from build123d import *

# Parameters (mm, degrees)
ESQUISSE1_W             = 100
ESQUISSE1_H             = 130
BOSS_EXTRU_1_DEPTH      = 6
ESQUISSE2_W             = 6
ESQUISSE2_H             = 30
ENL_V_MAT_EXTRU_1_DEPTH = 6


with BuildPart() as part:
    # Esquisse1 → Boss.-Extru.1 (new body)
    with BuildSketch(Plane.XY):
        with Locations((-50, 65)):
            Rectangle(ESQUISSE1_W, ESQUISSE1_H)
    extrude(amount=BOSS_EXTRU_1_DEPTH)

    # Esquisse2 → Enlèv. mat.-Extru.1 (cut)
    with BuildSketch(Plane.XY.offset(6)):
        Polygon((-100, 130), (-70, 130), (-70, 124), (-94, 124), (-94, 100), (-100, 100), align=None)
        Polygon((0, 130), (-30.235491659, 130), (-30.235491659, 124), (-6.235491659, 124), (-6.235491659, 100), (0, 100), align=None)
        Polygon((-100, 0), (-70, 0), (-70, 6), (-94, 6), (-94, 30), (-100, 30), align=None)
        Polygon((0, 0), (-30, 0), (-30, 6), (-6, 6), (-6, 30), (0, 30), align=None)
        with Locations((-97, 65)):
            Rectangle(ESQUISSE2_W, ESQUISSE2_H)
        with Locations((-3, 65)):
            Rectangle(ESQUISSE2_W, ESQUISSE2_H)
    extrude(amount=-ENL_V_MAT_EXTRU_1_DEPTH, mode=Mode.SUBTRACT)


solid = part.part
Read the model definition and answer for the solid it produces. Units are mm, in the model's axes. A direction names the side the tool comes from. Round coordinates to 2 decimals unless told otherwise and drop trailing zeros. Write each loop counter-clockwise with the first axis right and the second up, starting at its lowest first coordinate (ties: lowest second). Pieces come first, ordered by that corner, then holes. Notation, with made-up numbers: M 85.5,-20.5 L 134.5,-20.5 A15 ccw 134.5,-5.5 Z; hole C 5.5,65 d5. An arc over 180 degrees is marked long. Use a Markdown table: item, result.
1) Straight lines are drawn through the part: line 1 along Y through (x, z) = (-87, 4.15); line 2 along X through (y, z) = (108, 4.35); line 3 along X through (y, z) = (23.5, 5). For each, find the intervals that lie inside material, in ascending order. Write a range as [from, to].
Answers follow:
| item | result |
|---|---|
| line 1 | y = [6, 124] |
| line 2 | x = [-94, -6.24] |
| line 3 | x = [-94, -6] |
2) Flat-ended cylindrical pins translate along their axes: pin 1 (1.8 mm diameter, centred on x = -4.5, z = 3, fed in from -Y); pin 2 (1.8 mm diameter, centred on x = -21, z = 2.5, fed in from +Y); pin 3 (8 mm diameter, centred on x = -88.5, y = 63, fed in from -Z); pin 4 (1.8 mm diameter, centred on y = 107.5, z = 2.5, fed in from -X). Find the tip coordinate at first contact, or state that the pin passes through.
Answers follow:
| item | result |
|---|---|
| pin 1 | stops at y = 30 |
| pin 2 | stops at y = 124 |
| pin 3 | stops at z = 0 |
| pin 4 | stops at x = -94 |
3) For a pull along Y with two mould halves and no side action, classify faces 4 (the flat face through (0, 40, 3)), 5 (the flat face through (-18, 6, 3)), 6 (the flat face through (-6, 65, 3)) as pulls with the +Y half, pulls with the -Y half, needs draft (parallel to the pull), parting line crosses it, or undercut.
Answers follow:
| item | result |
|---|---|
| face 4 | needs draft |
| face 5 | pulls with the -Y half |
| face 6 | undercut |
4) The part is cut by section A-A (z = 4.5). Write down the section's boundary in (x, y).
Answers follow:
| item | result |
|---|---|
| outline | M -100,30 L -94,30 L -94,6 L -70,6 L -70,0 L -30,0 L -30,6 L -6,6 L -6,30 L 0,30 L 0,50 L -6,50 L -6,80 L 0,80 L 0,100 L -6.24,100 L -6.24,124 L -30.24,124 L -30.24,130 L -70,130 L -70,124 L -94,124 L -94,100 L -100,100 L -100,80 L -94,80 L -94,50 L -100,50 Z |
5) The part is cut by section C-C (x = -22.5). Write down the section's boundary in (y, z).
Answers follow:
| item | result |
|---|---|
| outline | M 6,0 L 124,0 L 124,6 L 6,6 Z |
6) The part is cut by section B-B (y = 52). Write down the section's boundary in (x, z).
Answers follow:
| item | result |
|---|---|
| outline | M -94,0 L -6,0 L -6,6 L -94,6 Z |
7) A tool of negligible diameter and unlimited length cuts with its end or side. For faces 1 (the flat face through (-30, 3, 3)), 2 (the flat face through (-30.235, 127, 3)), 3 (the flat face through (-82, 124, 3)), from which of +Z, -Z, +X, -X, +Y, -Y can it reach the whole face along a straight path? Write none if from no direction.
Answers follow:
| item | result |
|---|---|
| face 1 | +Z, -Z, +X, -Y |
| face 2 | +Z, -Z, +X, +Y |
| face 3 | +Z, -Z, -X, +Y |
